from build123d import *

# Parameters (mm, degrees)
SKETCH1_W              = 120
SKETCH1_H              = 15
SKETCH1_W_2            = 110
SKETCH1_H_2            = 5
SLIDER_MAIN_BODY_DEPTH = 5
SKETCH2_W              = 1.666666666
SKETCH2_H              = 5
TRACK_SLIDER_DEPTH     = 1.666666667
SKETCH3_W              = 5
SKETCH3_H              = 15
HANDLE_DEPTH           = 5
SKETCH5_W              = 105
SKETCH5_H              = 1.666666666
CUT_EXTRUDE1_DEPTH     = 67.895440801


with BuildPart() as part:
    # Sketch1 → Slider Main Body (new body)
    with BuildSketch(Plane.XY):
        Rectangle(SKETCH1_W, SKETCH1_H)
        Rectangle(SKETCH1_W_2, SKETCH1_H_2, mode=Mode.SUBTRACT)
    extrude(amount=SLIDER_MAIN_BODY_DEPTH)

    # Sketch2 → Track Slider (add)
    with BuildSketch(Plane.XZ.offset(7.5)):
        with Locations((-57.5, 2.5)):
            Rectangle(SKETCH2_W, SKETCH2_H)
    extrude(amount=TRACK_SLIDER_DEPTH)

    # Sketch3 → Handle (add)
    with BuildSketch(Plane.XY.offset(5)):
        with Locations((-62.5, 0)):
            Rectangle(SKETCH3_W, SKETCH3_H)
    extrude(amount=-HANDLE_DEPTH)

    # Sketch5 → Cut-Extrude1 (cut, through all)
    with BuildSketch(Plane.XZ.offset(7.5)):
        with Locations((-2.5, 2.5)):
            Rectangle(SKETCH5_W, SKETCH5_H)
    extrude(amount=-CUT_EXTRUDE1_DEPTH, mode=Mode.SUBTRACT)


solid = part.part
Part model, mm, in its own coordinate system. A direction names the side the tool comes from. Give positions to 0.01 mm unless a question says otherwise; leave off trailing zeros. Loops run counter-clockwise (first coordinate to the right, second up) from the corner with the lowest first, then second, coordinate; pieces in that order, holes last. Notation, with made-up numbers: M 59,67.5 L 117,67.5 A16 ccw 117,71.5 Z; hole C 49,80 d2. An arc over 180 degrees is marked long. Put each result on its own line as item: value. Start each with the question number.
1) Saw through at A-A (y = -3.75). List the corners of the cut face in (x, z).
2) Probe probe 1 along Y at (x, z) = (-12, 4.25); probe 2 along Z at (x, y) = (-34, 5.5); probe 3 along X at (y, z) = (-2, 3.65). List the from-to ranges inside material, lowest first.
3) Saw through at B-B (z = 4.2). List the corners of the cut face in (x, y).
4) Flat gauge pins, fed straight in: pin 1 (2.5 mm diameter, centred on x = 2, z = 1.5, fed in from -Y); pin 2 (0.5 mm diameter, centred on y = -8, z = 3.5, fed in from +X). Where does each tip first touch, or does it go through?
5) Pull direction Z, two halves, no side cores. Call faces 4 (the flat face through (-3, 5, 1.667)), 5 (the flat face through (-62, -7.5, 3)), 6 (the flat face through (-3, 3, 0)): +Z half, -Z half, draft (parallel to the pull), parting line (faces both ways), or undercut.
6) Saw through at C-C (x = -4). List the corners of the cut face in (y, z), then the cut area to 3 significant figures.
7) 3-axis set-ups, long thin cutter, end or side, ignore diameter. For faces 1 (the flat face through (55, 0, 2)), 2 (the flat face through (1, -7.5, 1)), 3 (the flat face through (-3, -5, 3.333)): which of +Z, -Z, +X, -X, +Y, -Y reach the whole face in a straight line?
Numbers:
1. outline: M -65,0 L 60,0 L 60,5 L -65,5 Z; hole M -55,1.67 L 50,1.67 L 50,3.33 L -55,3.33 Z
2. probe 1: -7.5 to -2.5, 2.5 to 7.5
2. probe 2: 0 to 1.67, 3.33 to 5
2. probe 3: -65 to -55, 55 to 60
3. outline: M -65,-7.5 L -58.33,-7.5 L -58.33,-9.17 L -56.67,-9.17 L -56.67,-7.5 L 60,-7.5 L 60,7.5 L -65,7.5 Z; hole M -55,-2.5 L 55,-2.5 L 55,2.5 L -55,2.5 Z
4. pin 1: y = -7.5
4. pin 2: x = -56.67
5. face 4: undercut
5. face 5: draft
5. face 6: -Z half
6. outline: M -7.5,0 L -2.5,0 L -2.5,1.67 L -7.5,1.67 Z; M -7.5,3.33 L -2.5,3.33 L -2.5,5 L -7.5,5 Z; M 2.5,0 L 7.5,0 L 7.5,1.67 L 2.5,1.67 Z; M 2.5,3.33 L 7.5,3.33 L 7.5,5 L 2.5,5 Z
6. area: 33.3 mm^2
7. face 1: +Z, -Z
7. face 2: +Z, -Z, +X, -Y
7. face 3: +Y, -Y
